from build123d import *

# Parameters (mm, degrees)
ESQUISSE1_W        = 20
ESQUISSE1_H        = 20
BOSS_EXTRU_1_DEPTH = 20
BOSS_EXTRU_2_DEPTH = 30
BOSS_EXTRU_3_DEPTH = 30
BOSS_EXTRU_4_DEPTH = 30
BOSS_EXTRU_5_DEPTH = 30
BOSS_EXTRU_6_DEPTH = 30
BOSS_EXTRU_7_DEPTH = 30


with BuildPart() as part:
    # Esquisse1 → Boss.-Extru.1 (new body)
    with BuildSketch(Plane.XY):
        with Locations((-38.912352392, 11.232287948)):
            Rectangle(ESQUISSE1_W, ESQUISSE1_H)
    extrude(amount=BOSS_EXTRU_1_DEPTH)

    # Esquisse2 → Boss.-Extru.2 (add)
    with BuildSketch(Plane.XY.offset(20)):
        Polygon((-41.362352392, 1.232287948), (-41.362352392, 2.782287948), (-45.062352392, 2.782287948), (-45.062352392, 3.782287948), (-41.562352392, 7.436545738), (-36.262352392, 7.436545738), (-32.762352392, 3.782287948), (-32.762352392, 2.782287948), (-36.462352392, 2.782287948), (-36.462352392, 1.232287948), align=None)
    extrude(amount=BOSS_EXTRU_2_DEPTH)

    # Esquisse3 → Boss.-Extru.3 (add)
    with BuildSketch(Plane(origin=(-28.912352392, 0, 0), x_dir=(0, 0, -1), z_dir=(1, 0, 0))):
        Polygon((0, 8.782287948), (-1.55, 8.782287948), (-1.55, 5.082287948), (-2.55, 5.082287948), (-6.204257791, 8.582287948), (-6.204257791, 13.882287948), (-2.55, 17.382287948), (-1.55, 17.382287948), (-1.55, 13.682287948), (0, 13.682287948), align=None)
    extrude(amount=BOSS_EXTRU_3_DEPTH)

    # Esquisse4 → Boss.-Extru.4 (add)
    with BuildSketch(Plane(origin=(0, 21.232287948, 0), x_dir=(1, 0, 0), z_dir=(0, 1, 0))):
        Polygon((-36.462352392, 0), (-36.462352392, -1.55), (-32.762352392, -1.55), (-32.762352392, -2.55), (-36.262352392, -6.204257791), (-41.562352392, -6.204257791), (-45.062352392, -2.55), (-45.062352392, -1.55), (-41.362352392, -1.55), (-41.362352392, 0), align=None)
    extrude(amount=BOSS_EXTRU_4_DEPTH)

    # Esquisse6 → Boss.-Extru.5 (add)
    with BuildSketch(Plane(origin=(-28.912352392, 0, 0), x_dir=(0, 0, -1), z_dir=(1, 0, 0))):
        Polygon((-12.45, 1.232287948), (-12.45, 2.782287948), (-16.15, 2.782287948), (-16.15, 3.782287948), (-12.65, 7.436545738), (-7.35, 7.436545738), (-3.85, 3.782287948), (-3.85, 2.782287948), (-7.55, 2.782287948), (-7.55, 1.232287948), align=None)
    extrude(amount=BOSS_EXTRU_5_DEPTH)

    # Esquisse8 → Boss.-Extru.6 (add)
    with BuildSketch(Plane(origin=(0, 21.232287948, 0), x_dir=(1, 0, 0), z_dir=(0, 1, 0))):
        Polygon((-48.912352392, -7.55), (-47.362352392, -7.55), (-47.362352392, -3.85), (-46.362352392, -3.85), (-42.708094601, -7.35), (-42.708094601, -12.65), (-46.362352392, -16.15), (-47.362352392, -16.15), (-47.362352392, -12.45), (-48.912352392, -12.45), align=None)
    extrude(amount=BOSS_EXTRU_6_DEPTH)

    # Esquisse9 → Boss.-Extru.7 (add)
    with BuildSketch(Plane.XY.offset(20)):
        Polygon((-48.912352392, 13.682287948), (-47.362352392, 13.682287948), (-47.362352392, 17.382287948), (-46.362352392, 17.382287948), (-42.708094601, 13.882287948), (-42.708094601, 8.582287948), (-46.362352392, 5.082287948), (-47.362352392, 5.082287948), (-47.362352392, 8.782287948), (-48.912352392, 8.782287948), align=None)
    extrude(amount=BOSS_EXTRU_7_DEPTH)


solid = part.part
Geometry: final body of the model. Coordinates: model frame, mm. A direction names the side the tool comes from. Round coordinates to 2 decimals unless told otherwise and drop trailing zeros. Loops run counter-clockwise (first coordinate to the right, second up) from the corner with the lowest first, then second, coordinate; pieces in that order, holes last.
Q1. Pull-direction query (X, two-part tool) for faces 5 (the flat face through (1.088, 11, 3)), 6 (the flat face through (-43.34, 5.58, 34.79)), 7 (the flat face through (-14, 13.682, 1)); classes: released by +X, released by -X, zero draft, split by the parting line, or undercut.
Q2. Section D-D on x = -40.5. Return loops of the section in (y, z).
Q3. Section B-B on z = 21.5. Return loops of the section in (x, y), plus the area to 3 significant figures.
Q4. Pin query (flat end, axial travel): P1, Ø6, axis at x = -22.5, z = 15, coming from the +Y side; P2, Ø0.5, axis at y = 2.5, z = 29, coming from the -X side; P3, Ø0.8, axis at x = -21, z = 2.5, coming from the +Y side. Return the tip coordinate at first contact, or that it passes through.
Q5. Section C-C on y = 9.5. Return loops of the section in (x, z), plus the area to 3 significant figures.
Q6. Material intervals for L1, parallel to X at y = 34.5, z = 2; L2, parallel to Z at x = -40.5, y = 46; L3, parallel to X at y = 7, z = 48.5, sorted ascending.
Q7. Access query for faces 1 (the flat face through (-47.362, 36, 6)), 2 (the flat face through (-44.561, 15.657, 34.79)), 3 (the flat face through (-14, 2.782, 6)), 4 (the flat face through (-47.362, 16, 35)). Directions: +Z, -Z, +X, -X, +Y, -Y. A direction counts if a zero-diameter tool reaches every point of the face in a straight line with its end or side. Return the directions, or none.
Q8. Section A-A on x = -20. Return loops of the section in (y, z).
Evaluation:
1. face 5: released by +X
1. face 6: undercut
1. face 7: zero draft
2. outline: (1.23, 0) - (51.23, 0) - (51.23, 6.2) - (21.23, 6.2) - (21.23, 20) - (7.44, 20) - (7.44, 50) - (1.23, 50) - close
3. outline: (-48.91, 8.78) - (-47.36, 8.78) - (-47.36, 5.08) - (-46.36, 5.08) - (-42.71, 8.58) - (-42.71, 13.88) - (-46.36, 17.38) - (-47.36, 17.38) - (-47.36, 13.68) - (-48.91, 13.68) - close; (-45.06, 2.78) - (-41.36, 2.78) - (-41.36, 1.23) - (-36.46, 1.23) - (-36.46, 2.78) - (-32.76, 2.78) - (-32.76, 3.78) - (-36.26, 7.44) - (-41.56, 7.44) - (-45.06, 3.78) - close
3. area: 104 mm2
4. P1: stops at y = 7.44
4. P2: stops at x = -41.36
4. P3: stops at y = 17.38
5. outline: (-48.91, 0) - (1.09, 0) - (1.09, 6.2) - (-28.91, 6.2) - (-28.91, 20) - (-42.71, 20) - (-42.71, 50) - (-48.91, 50) - close
5. area: 772 mm2
6. L1: x = -45.06 to -32.76
6. L2: z = 0 to 6.2
6. L3: x = -47.36 to -44.36, -41.98 to -35.84
7. face 1: -Z, -X, +Y
7. face 2: +Z, +X, +Y
7. face 3: -Z, +X, -Y
7. face 4: +Z, -X, +Y
8. outline: (1.23, 7.55) - (2.78, 7.55) - (2.78, 3.85) - (3.78, 3.85) - (7.44, 7.35) - (7.44, 12.65) - (3.78, 16.15) - (2.78, 16.15) - (2.78, 12.45) - (1.23, 12.45) - close; (5.08, 1.55) - (8.78, 1.55) - (8.78, 0) - (13.68, 0) - (13.68, 1.55) - (17.38, 1.55) - (17.38, 2.55) - (13.88, 6.2) - (8.58, 6.2) - (5.08, 2.55) - close
